```python
from build123d import *

# Parameters (mm, degrees)
EXTRUDE_1_DEPTH           = 215
SKETCH_2_R                = 12.5
EXTRUDE_2_DEPTH           = 10
EXTRUDE_2_DRAFT           = 15
EXTRUDE_2_PROFILE_2_DEPTH = 10
EXTRUDE_2_PROFILE_2_DRAFT = 15
EXTRUDE_2_PROFILE_3_DEPTH = 10
EXTRUDE_2_PROFILE_3_DRAFT = 15
EXTRUDE_2_PROFILE_4_DEPTH = 10
EXTRUDE_2_PROFILE_4_DRAFT = 15
SKETCH1_R                 = 11.40437452
BOSS_EXTRUDE1_DEPTH       = 20


with BuildPart() as part:
    # 草圖1 → 填料-伸長1 (new body)
    with BuildSketch(Plane.XY):
        with BuildLine():
            Line((-130.808640264, -66.769197125), (-91.433640264, 3.230802875))
            ThreePointArc((-91.433640264, 3.230802875), (-89.599992065, 5.095544116), (-87.075762578, 5.779496677))
            Line((-87.075762578, 5.779496677), (87.075762578, 5.779496677))
            ThreePointArc((87.075762578, 5.779496677), (89.599992065, 5.095544116), (91.433640264, 3.230802875))
            Line((91.433640264, 3.230802875), (130.808640264, -66.769197125))
            ThreePointArc((130.808640264, -66.769197125), (130.766810017, -71.74473281), (126.450762578, -74.220503323))
            Line((126.450762578, -74.220503323), (-126.450762578, -74.220503323))
            ThreePointArc((-126.450762578, -74.220503323), (-130.766810017, -71.74473281), (-130.808640264, -66.769197125))
        make_face()
    extrude(amount=EXTRUDE_1_DEPTH)


with BuildPart() as extrude_2_tool:
    # 草圖2 → 填料-伸長2 (with draft: the straight prism first)
    with BuildSketch(Plane.XZ.offset(74.220503323)):
        with Locations((-100, 185.989670211)):
            Circle(SKETCH_2_R)
    extrude(amount=EXTRUDE_2_DEPTH)
    # 填料-伸長2: the draft: its side faces are tilted about the plane it starts from
    extrude_2_sides = [extrude_2_tool.faces().sort_by_distance(p)[0] for p in [
        (-112.5, -79.220503323, 185.989670211),
    ]]
    draft(extrude_2_sides, Plane.XZ.offset(74.220503323), EXTRUDE_2_DRAFT)


with BuildPart() as part_1:
    add(part.part)

    # 填料-伸長2: add extrude_2_tool
    add(extrude_2_tool.part)


with BuildPart() as extrude_2_profile_2_tool:
    # 草圖2 → 填料-伸長2 profile 2 (with draft: the straight prism first)
    with BuildSketch(Plane.XZ.offset(74.220503323)):
        with Locations((-100, 29.010329789)):
            Circle(SKETCH_2_R)
    extrude(amount=EXTRUDE_2_PROFILE_2_DEPTH)
    # 填料-伸長2 profile 2: the draft: its side faces are tilted about the plane it starts from
    extrude_2_profile_2_sides = [extrude_2_profile_2_tool.faces().sort_by_distance(p)[0] for p in [
        (-112.5, -79.220503323, 29.010329789),
    ]]
    draft(extrude_2_profile_2_sides, Plane.XZ.offset(74.220503323), EXTRUDE_2_PROFILE_2_DRAFT)


with BuildPart() as part_2:
    add(part_1.part)

    # 填料-伸長2 profile 2: add extrude_2_profile_2_tool
    add(extrude_2_profile_2_tool.part)


with BuildPart() as extrude_2_profile_3_tool:
    # 草圖2 → 填料-伸長2 profile 3 (with draft: the straight prism first)
    with BuildSketch(Plane.XZ.offset(74.220503323)):
        with Locations((100, 29.010329789)):
            Circle(SKETCH_2_R)
    extrude(amount=EXTRUDE_2_PROFILE_3_DEPTH)
    # 填料-伸長2 profile 3: the draft: its side faces are tilted about the plane it starts from
    extrude_2_profile_3_sides = [extrude_2_profile_3_tool.faces().sort_by_distance(p)[0] for p in [
        (87.5, -79.220503323, 29.010329789),
    ]]
    draft(extrude_2_profile_3_sides, Plane.XZ.offset(74.220503323), EXTRUDE_2_PROFILE_3_DRAFT)


with BuildPart() as part_3:
    add(part_2.part)

    # 填料-伸長2 profile 3: add extrude_2_profile_3_tool
    add(extrude_2_profile_3_tool.part)


with BuildPart() as extrude_2_profile_4_tool:
    # 草圖2 → 填料-伸長2 profile 4 (with draft: the straight prism first)
    with BuildSketch(Plane.XZ.offset(74.220503323)):
        with Locations((100, 185.989670211)):
            Circle(SKETCH_2_R)
    extrude(amount=EXTRUDE_2_PROFILE_4_DEPTH)
    # 填料-伸長2 profile 4: the draft: its side faces are tilted about the plane it starts from
    extrude_2_profile_4_sides = [extrude_2_profile_4_tool.faces().sort_by_distance(p)[0] for p in [
        (87.5, -79.220503323, 185.989670211),
    ]]
    draft(extrude_2_profile_4_sides, Plane.XZ.offset(74.220503323), EXTRUDE_2_PROFILE_4_DRAFT)


with BuildPart() as part_4:
    add(part_3.part)

    # 填料-伸長2 profile 4: add extrude_2_profile_4_tool
    add(extrude_2_profile_4_tool.part)

    # Sketch1 → Boss-Extrude1 (add)
    with BuildSketch(Plane(origin=(0, 5.779496677, 0), x_dir=(1, 0, 0), z_dir=(0, 1, 0))):
        with Locations(Location((1.433640264, -185, 0), (0, 0, 270))):
            Circle(SKETCH1_R)
    extrude(amount=BOSS_EXTRUDE1_DEPTH)


solid = part_4.part
```
Input: part model. Units: mm. Frame: model coordinates. A direction names the side the tool comes from. Coordinates: 2 decimals unless noted, no trailing zeros. Order: outer loops, then holes, each group sorted by start corner. A loop starts at its lowest first (then second) coordinate and runs counter-clockwise, first axis right, second up. Notation, with made-up numbers: (56, 38) - (105, 38) arc R18 cw to (105, 53) - close; hole circle Ø1 at (-11, 73). An arc over 180 degrees is marked (long way). Return JSON: item names as keys, results as strings.
Q1. Ray query, probe 1 along Y at (x, z) = (27, 136.5); probe 2 along Z at (x, y) = (93.5, -77.5); probe 3 along X at (y, z) = (-76, 18). Return the intervals inside material, ascending.
The answers:
{"probe 1": "y = -74.22 to 5.78", "probe 2": "z = 19.38 to 38.64, 176.36 to 195.62", "probe 3": "x = -104.83 to -95.17, 95.17 to 104.83"}
Q2. Cut plane B-B (x = -100). Return loops of the section in (y, z), then the cut area to 3 significant figures.
The answers:
{"outline": "(-84.22, 19.19) - (-74.22, 16.51) - (-74.22, 0) - (-12, 0) - (-12, 215) - (-74.22, 215) - (-74.22, 198.49) - (-84.22, 195.81) - (-84.22, 176.17) - (-74.22, 173.49) - (-74.22, 41.51) - (-84.22, 38.83) - close", "area": "13,800 mm2"}
Q3. Cut plane C-C (y = -48.5). Return loops of the section in (x, z).
The answers:
{"outline": "(-120.53, 0) - (120.53, 0) - (120.53, 215) - (-120.53, 215) - close"}
Q4. First-contact query: pin 1 (8 mm diameter, centred on y = -6, z = 60.5, fed in from -X); pin 2 (6 mm diameter, centred on y = -66, z = 71, fed in from +X); pin 3 (8 mm diameter, centred on x = -19.5, z = 114, fed in from -Y). Flat tips, straight axial feed; report the tip coordinate or a pass-through.
The answers:
{"pin 1": "stops at x = -98.88", "pin 2": "stops at x = 131.45", "pin 3": "stops at y = -74.22"}
Q5. Cut plane A-A (z = 113.5). Return loops of the section in (x, y), then the cut area to 3 significant figures.
The answers:
{"outline": "(-130.81, -66.77) arc R5 ccw to (-126.45, -74.22) - (126.45, -74.22) arc R5 ccw to (130.81, -66.77) - (91.43, 3.23) arc R5 ccw to (87.08, 5.78) - (-87.08, 5.78) arc R5 ccw to (-91.43, 3.23) - close", "area": "18,000 mm2"}
Q6. Cut plane D-D (x = -33). Return loops of the section in (y, z), then the cut area to 3 significant figures.
The answers:
{"outline": "(-74.22, 0) - (5.78, 0) - (5.78, 215) - (-74.22, 215) - close", "area": "17,200 mm2"}
Q7. Access query for faces 1 (the cylindrical face through (1.935, 15.639, 173.607)), 2 (the flat face through (100, -84.221, 186)). Directions: +Z, -Z, +X, -X, +Y, -Y. A direction counts if a zero-diameter tool reaches every point of the face in a straight line with its end or side. Return the directions, or none.
The answers:
{"face 1": "+Y", "face 2": "+Z, -Z, +X, -X, -Y"}
Q8. Draft query along Z for faces 3 (the flat face through (100, -84.221, 29)), 4 (the conical face through (-102.23, -82.48, 18.97)), 5 (the flat face through (2, -34, 0)). Return one class per face: +Z half, -Z half, draft (parallel to the pull), parting line (faces both ways), or undercut.
The answers:
{"face 3": "draft", "face 4": "undercut", "face 5": "-Z half"}
